```python
from build123d import *

# Parameters (mm, degrees)
SKETCH1_R           = 35
SKETCH1_R_2         = 17.5
BOSS_EXTRUDE1_DEPTH = 5
SKETCH2_R           = 30
SKETCH2_R_2         = 22
SKETCH2_R_3         = 1.6
BOSS_EXTRUDE2_DEPTH = 5
SKETCH3_R           = 1.5
CUT_EXTRUDE1_DEPTH  = 5
SKETCH4_R           = 26
CUT_EXTRUDE2_DEPTH  = 2.5


with BuildPart() as part:
    # Sketch1 → Boss-Extrude1 (new body)
    with BuildSketch(Plane(origin=(0, 0, 0), x_dir=(1, 0, 0), z_dir=(0, 1, 0))):
        with Locations(Location((0, 0, 0), (0, 0, 270))):
            Circle(SKETCH1_R)
        with Locations(Location((0, 0, 0), (0, 0, 270))):
            Circle(SKETCH1_R_2, mode=Mode.SUBTRACT)
    extrude(amount=BOSS_EXTRUDE1_DEPTH)

    # Sketch2 → Boss-Extrude2 (add)
    with BuildSketch(Plane.XZ):
        with Locations(Location((0, 0, 0), (0, 0, 90))):
            Circle(SKETCH2_R)
        with Locations(Location((0, 0, 0), (0, 0, 270))):
            Circle(SKETCH2_R_2, mode=Mode.SUBTRACT)
        with Locations(Location((0, 27.5, 0), (0, 0, 270))):
            Circle(SKETCH2_R_3, mode=Mode.SUBTRACT)
        with Locations(Location((5.535709302, 26.937073384, 0), (0, 0, 270))):
            Circle(SKETCH2_R_3, mode=Mode.SUBTRACT)
        with Locations(Location((10.844786016, 25.27133982, 0), (0, 0, 270))):
            Circle(SKETCH2_R_3, mode=Mode.SUBTRACT)
        with Locations(Location((15.709875915, 22.570994633, 0), (0, 0, 270))):
            Circle(SKETCH2_R_3, mode=Mode.SUBTRACT)
        with Locations(Location((19.931801649, 18.946590275, 0), (0, 0, 270))):
            Circle(SKETCH2_R_3, mode=Mode.SUBTRACT)
        with Locations(Location((23.337717081, 14.546510284, 0), (0, 0, 270))):
            Circle(SKETCH2_R_3, mode=Mode.SUBTRACT)
        with Locations(Location((25.788183634, 9.550894453, 0), (0, 0, 270))):
            Circle(SKETCH2_R_3, mode=Mode.SUBTRACT)
        with Locations(Location((27.182878919, 4.164263881, 0), (0, 0, 270))):
            Circle(SKETCH2_R_3, mode=Mode.SUBTRACT)
        with Locations(Location((27.464703947, -1.392852143, 0), (0, 0, 270))):
            Circle(SKETCH2_R_3, mode=Mode.SUBTRACT)
        with Locations(Location((26.622120769, -6.892944637, 0), (0, 0, 270))):
            Circle(SKETCH2_R_3, mode=Mode.SUBTRACT)
        with Locations(Location((24.689624838, -12.110839168, 0), (0, 0, 270))):
            Circle(SKETCH2_R_3, mode=Mode.SUBTRACT)
        with Locations(Location((21.746332766, -16.83291452, 0), (0, 0, 270))):
            Circle(SKETCH2_R_3, mode=Mode.SUBTRACT)
        with Locations(Location((17.912743275, -20.865848374, 0), (0, 0, 270))):
            Circle(SKETCH2_R_3, mode=Mode.SUBTRACT)
        with Locations(Location((13.34580397, -24.044531944, 0), (0, 0, 270))):
            Circle(SKETCH2_R_3, mode=Mode.SUBTRACT)
        with Locations(Location((8.232485882, -26.238829551, 0), (0, 0, 270))):
            Circle(SKETCH2_R_3, mode=Mode.SUBTRACT)
        with Locations(Location((2.782128855, -27.358906393, 0), (0, 0, 270))):
            Circle(SKETCH2_R_3, mode=Mode.SUBTRACT)
        with Locations(Location((-2.782128855, -27.358906393, 0), (0, 0, 270))):
            Circle(SKETCH2_R_3, mode=Mode.SUBTRACT)
        with Locations(Location((-8.232485882, -26.238829551, 0), (0, 0, 270))):
            Circle(SKETCH2_R_3, mode=Mode.SUBTRACT)
        with Locations(Location((-13.34580397, -24.044531944, 0), (0, 0, 270))):
            Circle(SKETCH2_R_3, mode=Mode.SUBTRACT)
        with Locations(Location((-17.912743275, -20.865848374, 0), (0, 0, 270))):
            Circle(SKETCH2_R_3, mode=Mode.SUBTRACT)
        with Locations(Location((-21.746332766, -16.83291452, 0), (0, 0, 270))):
            Circle(SKETCH2_R_3, mode=Mode.SUBTRACT)
        with Locations(Location((-24.689624838, -12.110839168, 0), (0, 0, 270))):
            Circle(SKETCH2_R_3, mode=Mode.SUBTRACT)
        with Locations(Location((-26.622120769, -6.892944637, 0), (0, 0, 270))):
            Circle(SKETCH2_R_3, mode=Mode.SUBTRACT)
        with Locations(Location((-27.464703947, -1.392852143, 0), (0, 0, 270))):
            Circle(SKETCH2_R_3, mode=Mode.SUBTRACT)
        with Locations(Location((-27.182878919, 4.164263881, 0), (0, 0, 270))):
            Circle(SKETCH2_R_3, mode=Mode.SUBTRACT)
        with Locations(Location((-25.788183634, 9.550894453, 0), (0, 0, 270))):
            Circle(SKETCH2_R_3, mode=Mode.SUBTRACT)
        with Locations(Location((-23.337717081, 14.546510284, 0), (0, 0, 270))):
            Circle(SKETCH2_R_3, mode=Mode.SUBTRACT)
        with Locations(Location((-19.931801649, 18.946590275, 0), (0, 0, 270))):
            Circle(SKETCH2_R_3, mode=Mode.SUBTRACT)
        with Locations(Location((-15.709875915, 22.570994633, 0), (0, 0, 270))):
            Circle(SKETCH2_R_3, mode=Mode.SUBTRACT)
        with Locations(Location((-10.844786016, 25.27133982, 0), (0, 0, 270))):
            Circle(SKETCH2_R_3, mode=Mode.SUBTRACT)
        with Locations(Location((-5.535709302, 26.937073384, 0), (0, 0, 270))):
            Circle(SKETCH2_R_3, mode=Mode.SUBTRACT)
    extrude(amount=BOSS_EXTRUDE2_DEPTH)

    # Sketch3 → Cut-Extrude1 (cut)
    with BuildSketch(Plane(origin=(0, 5, 0), x_dir=(1, 0, 0), z_dir=(0, 1, 0))):
        with Locations(Location((0, 32.5, 0), (0, 0, 270))):
            Circle(SKETCH3_R)
        with Locations(Location((28.145825623, 16.25, 0), (0, 0, 270))):
            Circle(SKETCH3_R)
        with Locations(Location((28.145825623, -16.25, 0), (0, 0, 270))):
            Circle(SKETCH3_R)
        with Locations(Location((0, -32.5, 0), (0, 0, 270))):
            Circle(SKETCH3_R)
        with Locations(Location((-28.145825623, -16.25, 0), (0, 0, 270))):
            Circle(SKETCH3_R)
        with Locations(Location((-28.145825623, 16.25, 0), (0, 0, 270))):
            Circle(SKETCH3_R)
    extrude(amount=-CUT_EXTRUDE1_DEPTH, mode=Mode.SUBTRACT)

    # Sketch4 → Cut-Extrude2 (cut)
    with BuildSketch(Plane(origin=(0, 5, 0), x_dir=(1, 0, 0), z_dir=(0, 1, 0))):
        with Locations(Location((0, 0, 0), (0, 0, 270))):
            Circle(SKETCH4_R)
    extrude(amount=-CUT_EXTRUDE2_DEPTH, mode=Mode.SUBTRACT)


solid = part.part
```
Design review of the part built by this model. Coordinates are the model's own, in mm. A direction names the side the tool comes from. Round coordinates to 2 decimals unless told otherwise and drop trailing zeros. Order: outer loops, then holes, each group sorted by start corner. A loop starts at its lowest first (then second) coordinate and runs counter-clockwise, first axis right, second up. Notation, with made-up numbers: M -32.75,12 L -22.75,12 A30 ccw -22.75,36 Z; hole C -35.75,76 d4. An arc over 180 degrees is marked long. Put each result on its own line as item: value.
Q1. Insertion check: pin 1 Ø1 at (x, z) = (20.5, 18.5) entering from -Y; pin 2 Ø1.5 at (x, y) = (12.5, 1.5) entering from -Z; pin 3 Ø2 at (y, z) = (0, -19) entering from -X. Each pin has a flat end and moves straight along its axis. Give the tip position at first contact, or say it passes through.
Reported:
pin 1: y = 0
pin 2: z = -32.97
pin 3: x = -30.02
Q2. Machinability: for faces 1 (the face through (27, 0, -1)), 2 (the face through (-17, 2.5, 5)), 3 (the face through (-10.648, 1.232, -13.887)), which of the approach directions +Z, -Z, +X, -X, +Y, -Y give a long, thin tool a straight path to every point of the face, cutting with its end or side? Answer none if there is none.
Reported:
face 1: -Y
face 2: +Y
face 3: +Y, -Y
Q3. To check wall thickness, follow line 1 (Z direction, x = -13, y = -3); line 2 (Z direction, x = -27.5, y = -1); line 3 (Z direction, x = -14.5, y = -1). State the ranges of each line that lie inside material, in increasing order.
Reported:
line 1: -27.04 to -25.61, -22.48 to -17.75, 17.75 to 27.04
line 2: -11.99 to -8.23, -5.56 to -2.99, 0.21 to 2.6, 5.73 to 11.99
line 3: -26.26 to -25.15, -22.94 to -16.55, 16.55 to 21.52, 23.62 to 26.26
Q4. Consider section A-A (x = 0). State how many separate pieces and enclosed holes the cut face has, and give its area (4 significant figures).
Reported:
separate pieces: 4
enclosed holes: 0
area: 166.5 mm²
Q5. Draft analysis for pull direction Z (two halves, no side actions). For faces 4 (the face through (20, 0, 19)), 5 (the face through (18, -5, -13)), 6 (the face through (-21, 2, -28)), state which applies: released by +Z, released by -Z, zero draft, split by the parting line, or undercut.
Reported:
face 4: undercut
face 5: zero draft
face 6: split by the parting line
Q6. Consider section C-C (z = -32.5). State the section outline as (x, y) points, and give its area (3 significant figures).
Reported:
outline: M -12.99,0 L -1.5,0 L -1.5,5 L -12.99,5 Z; M 1.5,0 L 12.99,0 L 12.99,5 L 1.5,5 Z
area: 115 mm²
Q7. Consider section B-B (y = 3.5). State the section outline as (x, z) points, and give its area (3 significant figures).
Reported:
outline: C 0,0 d70; hole C -28.15,-16.25 d3; hole C -28.15,16.25 d3; hole C 0,0 d52; hole C 0,-32.5 d3; hole C 0,32.5 d3; hole C 28.15,-16.25 d3; hole C 28.15,16.25 d3
area: 1,680 mm²
